The drawing under review shows one solid part. Ordinate dimensions are in mm from its lowest x, y, z. A direction names the side the tool comes from. Round coordinates to 2 decimals unless told otherwise and drop trailing zeros. Loops run counter-clockwise (first coordinate to the right, second up) from the corner with the lowest first, then second, coordinate; pieces in that order, holes last. Notation, with made-up numbers: M 20,-39 L 55,-39 A18 cw 55,-7 Z; hole C 40,68.5 d1. An arc over 180 degrees is marked long. Use a Markdown table: item, result.
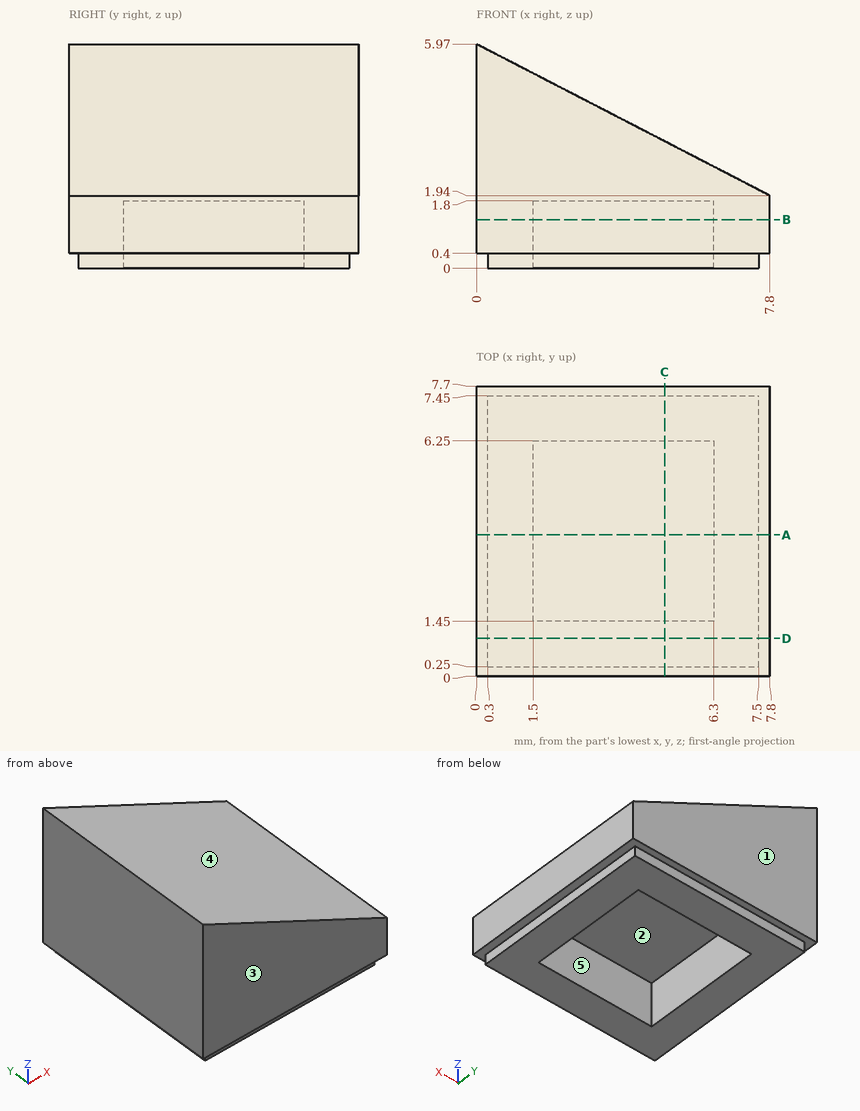
1. Take a section at D-D on y = 1. Give the boundary of the cut face in (x, z), and give its area (3 significant figures).
Check values:
| item | result |
|---|---|
| outline | M 0,0.4 L 0.3,0.4 L 0.3,0 L 7.5,0 L 7.5,0.4 L 7.8,0.4 L 7.8,1.94 L 0,5.97 Z |
| area | 30.6 mm² |
2. Machinability: for the marked faces 1 and 2, which of the approach directions +Z, -Z, +X, -X, +Y, -Y give a long, thin tool a straight path to every point of the face, cutting with its end or side? Answer none if there is none.
Check values:
| item | result |
|---|---|
| face 1 | +Z, -Z, +X, -X, +Y |
| face 2 | -Z |
3. Take a section at C-C on x = 5. Give the boundary of the cut face in (y, z), and give its area (3 significant figures).
Check values:
| item | result |
|---|---|
| outline | M 0,0.4 L 0.25,0.4 L 0.25,0 L 1.45,0 L 1.45,1.8 L 6.25,1.8 L 6.25,0 L 7.45,0 L 7.45,0.4 L 7.7,0.4 L 7.7,3.39 L 0,3.39 Z |
| area | 17.2 mm² |
4. Take a section at A-A on y = 3.75. Give the boundary of the cut face in (x, z).
Check values:
| item | result |
|---|---|
| outline | M 0,0.4 L 0.3,0.4 L 0.3,0 L 1.5,0 L 1.5,1.8 L 6.3,1.8 L 6.3,0 L 7.5,0 L 7.5,0.4 L 7.8,0.4 L 7.8,1.94 L 0,5.97 Z |
5. Take a section at B-B on z = 1.3. Give the boundary of the cut face in (x, y), and give its area (3 significant figures).
Check values:
| item | result |
|---|---|
| outline | M 0,0 L 7.8,0 L 7.8,7.7 L 0,7.7 Z; hole M 1.5,1.45 L 6.3,1.45 L 6.3,6.25 L 1.5,6.25 Z |
| area | 37.0 mm² |
6. Wall thickness on line 1 along X through (y, z) = (2, 1.75); line 2 along Y through (x, z) = (4.25, 1.05); line 3 along X through (y, z) = (6.25, 3.7): over which ranges is each line inside the solid? List them lowest first. Write a range as from..to.
Check values:
| item | result |
|---|---|
| line 1 | x = 0..1.5, 6.3..7.8 |
| line 2 | y = 0..1.45, 6.25..7.7 |
| line 3 | x = 0..4.39 |
7. The part is to be moulded in two halves that separate along Y. For the marked faces 3, 4 and 5, say which applies: pulls with the +Y half, pulls with the -Y half, needs draft (parallel to the pull), parting line crosses it, or undercut.
Check values:
| item | result |
|---|---|
| face 3 | pulls with the -Y half |
| face 4 | needs draft |
| face 5 | undercut |
8. Insertion check: pin 1 (1.4 mm diameter, centred on x = 4.5, y = 4.5, fed in from -Z); pin 2 (2 mm diameter, centred on y = 3.5, z = 4, fed in from +X); pin 3 (4 mm diameter, centred on x = 5, y = 4.5, fed in from +Z). Each pin has a flat end and moves straight along its axis. Give the tip position at first contact, or say it passes through.
Check values:
| item | result |
|---|---|
| pin 1 | stops at z = 1.8 |
| pin 2 | stops at x = 5.75 |
| pin 3 | stops at z = 4.42 |
